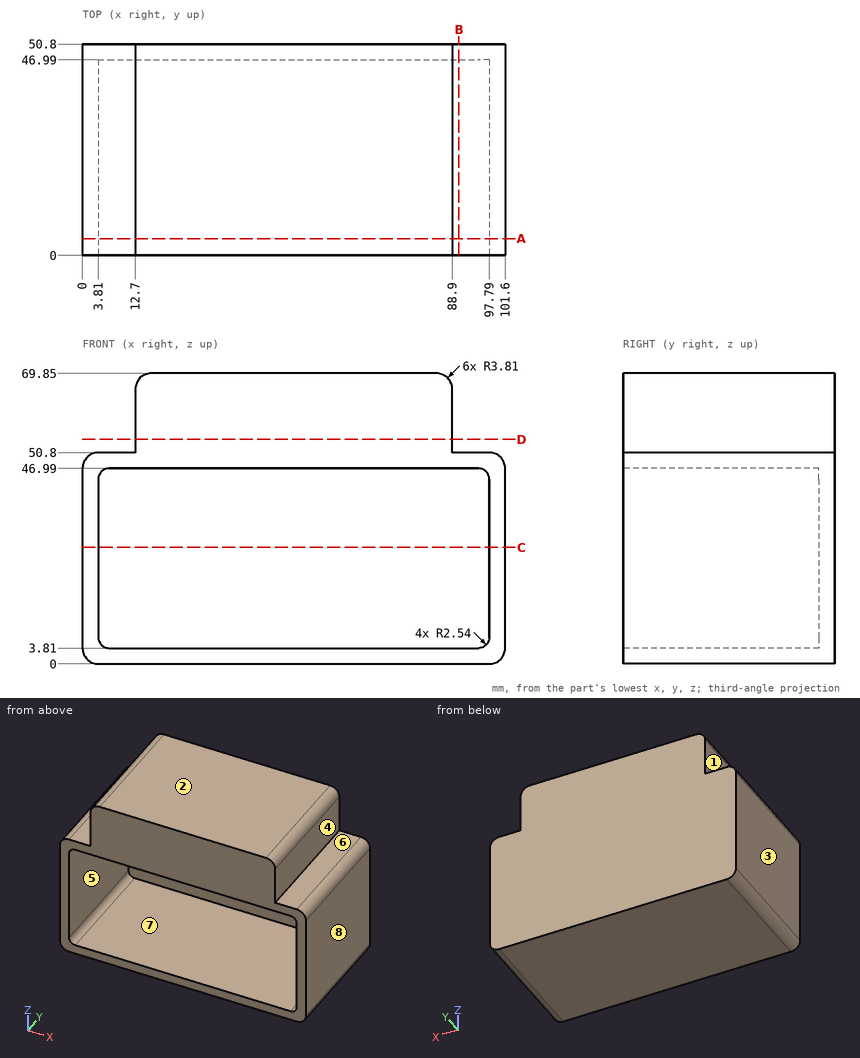
Geometry: see drawing. Coordinates: mm, zero at the bounding-box minimum. A direction names the side the tool comes from. Round coordinates to 2 decimals unless told otherwise and drop trailing zeros. Loops run counter-clockwise (first coordinate to the right, second up) from the corner with the lowest first, then second, coordinate; pieces in that order, holes last. Notation, with made-up numbers: (-5.75, -15) - (7.25, -15) arc R19 cw to (7.25, 14) - close; hole circle Ø1 at (-29.5, 37). An arc over 180 degrees is marked (long way). One line per item, written item: value. Start each with the question number.
(1) Ray query, line 1 (X direction, y = 46.5, z = 13.5); line 2 (Z direction, x = 61, y = 41); line 3 (Z direction, x = 89, y = 35). Return the intervals inside material, ascending. Write a range as [from, to].
(2) Section A-A, the plane y = 4. Return loops of the section in (x, z), plus the area to 3 significant figures.
(3) Access query for the marked faces 1, 2, 3, 4 and 5. Directions: +Z, -Z, +X, -X, +Y, -Y. A direction counts if a zero-diameter tool reaches every point of the face in a straight line with its end or side. Return the directions, or none.
(4) Contact query for flat-ended pins moving along their axis: P1, Ø1, axis at y = 38, z = 52, coming from the -X side; P2, Ø4.5, axis at x = 95, y = 34, coming from the +Z side; P3, Ø10, axis at x = 9, y = 20.5, coming from the +Z side. Output: stop coordinate, or through.
(5) Draft query along Z for the marked faces 6, 7 and 8. Return one class per face: +Z half, -Z half, draft (parallel to the pull), parting line (faces both ways), or undercut.
(6) Section C-C, the plane z = 28. Return loops of the section in (x, y), plus the area to 3 significant figures.
(7) Section D-D, the plane z = 54. Return loops of the section in (x, y).
(8) Section B-B, the plane x = 90.5. Return loops of the section in (y, z).
Results below:
1. line 1: [0, 3.81], [97.79, 101.6]
1. line 2: [0, 3.81], [46.99, 69.85]
1. line 3: [0, 3.81], [46.99, 50.8]
2. outline: (0, 3.81) arc R3.81 ccw to (3.81, 0) - (97.79, 0) arc R3.81 ccw to (101.6, 3.81) - (101.6, 46.99) arc R3.81 ccw to (97.79, 50.8) - (88.9, 50.8) - (88.9, 66.04) arc R3.81 ccw to (85.09, 69.85) - (16.51, 69.85) arc R3.81 ccw to (12.7, 66.04) - (12.7, 50.8) - (3.81, 50.8) arc R3.81 ccw to (0, 46.99) - close; hole (3.81, 6.35) arc R2.54 ccw to (6.35, 3.81) - (95.25, 3.81) arc R2.54 ccw to (97.79, 6.35) - (97.79, 44.45) arc R2.54 ccw to (95.25, 46.99) - (6.35, 46.99) arc R2.54 ccw to (3.81, 44.45) - close
2. area: 2,540 mm^2
3. face 1: +Z, -X, +Y, -Y
3. face 2: +Z, +X, -X, +Y, -Y
3. face 3: +Z, -Z, -X, +Y, -Y
3. face 4: +Z, +X, +Y, -Y
3. face 5: -Y
4. P1: x = 12.7
4. P2: z = 50.8
4. P3: z = 68.91
5. face 6: +Z half
5. face 7: undercut
5. face 8: draft
6. outline: (0, 0) - (3.81, 0) - (3.81, 46.99) - (97.79, 46.99) - (97.79, 0) - (101.6, 0) - (101.6, 50.8) - (0, 50.8) - close
6. area: 745 mm^2
7. outline: (12.7, 0) - (88.9, 0) - (88.9, 50.8) - (12.7, 50.8) - close
8. outline: (0, 0) - (50.8, 0) - (50.8, 50.8) - (0, 50.8) - (0, 46.99) - (46.99, 46.99) - (46.99, 3.81) - (0, 3.81) - close
